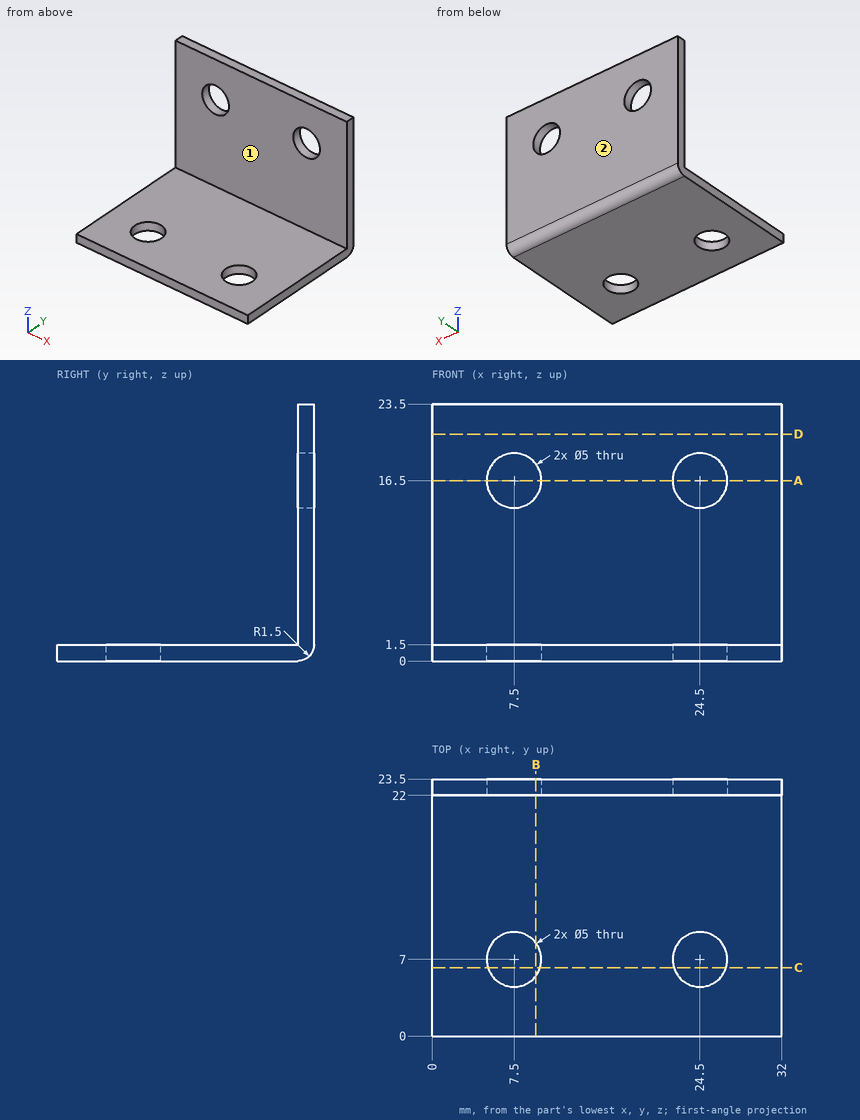
Part print with two shaded views. Sizes in mm from the minimum x, y, z corner. A direction names the side the tool comes from. Round coordinates to 2 decimals unless told otherwise and drop trailing zeros. Order: outer loops, then holes, each group sorted by start corner. A loop starts at its lowest first (then second) coordinate and runs counter-clockwise, first axis right, second up.
(1) Pin check, flat tips, straight feed: pin 1 (3 mm diameter, centred on x = 18, z = 5, fed in from -Y); pin 2 (4 mm diameter, centred on x = 24.5, z = 16.5, fed in from -Y); pin 3 (8 mm diameter, centred on x = 24.5, y = 7, fed in from +Z). Stop position of each tip, or through.
(2) 3-axis set-ups, long thin cutter, end or side, ignore diameter. For the marked faces 1 and 2: which of +Z, -Z, +X, -X, +Y, -Y reach the whole face in a straight line?
(3) Drill centre lines: line 1 (Z direction, x = 17.5, y = 18.75); line 2 (Y direction, x = 5.5, z = 22.5); line 3 (Y direction, x = 24.5, z = 0.85). Where is each one in solid material? Low to high.
(4) Band-saw the part on C-C (y = 6.25). List the corners of the cut face in (x, z).
(5) Band-saw the part on D-D (z = 20.75). List the corners of the cut face in (x, y).
(6) Band-saw the part on A-A (z = 16.5). List the corners of the cut face in (x, y), then the cut area to 3 significant figures.
(7) Band-saw the part on B-B (x = 9.5). List the corners of the cut face in (y, z), then the cut area to 3 significant figures.
Verdict:
1. pin 1: stops at y = 22
1. pin 2: passes through
1. pin 3: stops at z = 1.5
2. face 1: +Z, +X, -X, -Y
2. face 2: +Z, -Z, +X, -X, +Y
3. line 1: z = 0 to 1.5
3. line 2: y = 22 to 23.5
3. line 3: y = 0 to 4.5, 9.5 to 23.35
4. outline: (0, 0) - (5.12, 0) - (5.12, 1.5) - (0, 1.5) - close; (9.88, 0) - (22.12, 0) - (22.12, 1.5) - (9.88, 1.5) - close; (26.88, 0) - (32, 0) - (32, 1.5) - (26.88, 1.5) - close
5. outline: (0, 22) - (32, 22) - (32, 23.5) - (0, 23.5) - close
6. outline: (0, 22) - (5, 22) - (5, 23.5) - (0, 23.5) - close; (10, 22) - (22, 22) - (22, 23.5) - (10, 23.5) - close; (27, 22) - (32, 22) - (32, 23.5) - (27, 23.5) - close
6. area: 33.0 mm2
7. outline: (0, 0) - (5.5, 0) - (5.5, 1.5) - (0, 1.5) - close; (8.5, 0) - (22, 0) arc R1.5 ccw to (23.5, 1.5) - (23.5, 15) - (22, 15) - (22, 1.5) - (8.5, 1.5) - close; (22, 18) - (23.5, 18) - (23.5, 23.5) - (22, 23.5) - close
7. area: 58.8 mm2
